For this review, take the finished solid that the model builds, in its own axes (mm). A direction names the side the tool comes from. Round coordinates to 2 decimals unless told otherwise and drop trailing zeros. Order: outer loops, then holes, each group sorted by start corner. A loop starts at its lowest first (then second) coordinate and runs counter-clockwise, first axis right, second up. Notation, with made-up numbers: (30, 52) -> (43, 52) arc R28 cw to (43, 72) -> close; hole circle Ø5 at (16.25, 14.5). An arc over 180 degrees is marked (long way). Answer in a Markdown table with one row per item.
Autodesk Inventor part; units mm, degrees
ref_plane "YZ Plane" through (0, 0, 0) normal (1, 0, 0) x (0, 1, 0)
ref_plane "XZ Plane" through (0, 0, 0) normal (0, 1, 0) x (-1, 0, 0)
ref_plane "XY Plane" through (0, 0, 0) normal (0, 0, 1) x (1, 0, 0)
sketch "Esboço1" plane through (0, 0, 0) normal (0, 1, 0) x (-1, 0, 0)
  circle A0 centre (0, 0) radius 1.5
  dimension "d0" = 3
extrude "Extrusão1" add sketch "Esboço1" along normal blind 10.8
sketch "Esboço2" plane through (0, 10.8, 0) normal (0, 1, 0) x (1, 0, 0)
  circle A0 centre (0, 0) radius 1.5
  arc A1 (1.118, 1) -> (-1.118, 1) centre (0, 0) ccw
  line L0 (-1.118, 1) -> (1.118, 1)
  dimension "d3" = 0.5
extrude "Extrusão2" cut sketch "Esboço2" against normal blind 9 contours L0 A0 picked at (-0.0599, 1.1631)
sketch "Esboço3" plane through (0, 0, 0) normal (0, -1, 0) x (1, 0, 0)
  circle A0 centre (0, 0) radius 0.5
  dimension "d6" = 1
extrude "Extrusão3" add sketch "Esboço3" along normal blind 5
sketch "Esboço4" plane through (0, -5, 0) normal (0, -1, 0) x (1, 0, 0)
  circle A0 centre (0, 0) radius 0.6
  dimension "d9" = 1.2
extrude "Extrusão4" add sketch "Esboço4" along normal blind 0.2
fillet "Arredondamento1" radius 0.2 2 edges at (-1.4013, 10.8, -0.5352) (0.5352, 10.8, 1.4013)
properties part number "Eixo - Encaixe D"
Q1. Take a section at D-D, the plane y = 6.75. Write out the cut boundary in (x, z).
Answer key:
| item | result |
|---|---|
| outline | (-1.12, -1) -> (1.12, -1) arc R1.5 ccw (long way) to start |
Q2. Tool access review of faces 1 (the face through (0, 10.8, 0)), 2 (the face through (0, 6, -1)), 3 (the face through (-0.108, -2.465, 0.488)): name each direction out of +Z, -Z, +X, -X, +Y, -Y from which nothing blocks a thin tool from reaching the whole face with its end or side.
Answer key:
| item | result |
|---|---|
| face 1 | +Z, -Z, +X, -X, +Y |
| face 2 | -Z, +X, -X, +Y |
| face 3 | none |
Q3. Take a section at A-A, the plane z = 0. Write out the cut boundary in (x, y).
Answer key:
| item | result |
|---|---|
| outline | (-1.5, 0) -> (-0.5, 0) -> (-0.5, -5) -> (-0.6, -5) -> (-0.6, -5.2) -> (0.6, -5.2) -> (0.6, -5) -> (0.5, -5) -> (0.5, 0) -> (1.5, 0) -> (1.5, 10.6) arc R0.2 ccw to (1.3, 10.8) -> (-1.3, 10.8) arc R0.2 ccw to (-1.5, 10.6) -> close |
Q4. Clearance check with flat-ended pins moving along their axes: pin 1 Ø0.7 at (x, y) = (-0.5, 5) entering from -Z; pin 2 Ø1.5 at (x, y) = (0.5, -1.5) entering from -Z; pin 3 Ø1 at (y, z) = (7.5, -0.5) entering from +X. State where each tip first meets the part, or that it passes through.
Answer key:
| item | result |
|---|---|
| pin 1 | stops at z = -1 |
| pin 2 | stops at z = -0.5 |
| pin 3 | stops at x = 1.5 |
Q5. Take a section at B-B, the plane x = 0. Write out the cut boundary in (y, z), then the cut area to 3 significant figures.
Answer key:
| item | result |
|---|---|
| outline | (-5.2, -0.6) -> (-5, -0.6) -> (-5, -0.5) -> (0, -0.5) -> (0, -1.5) -> (1.8, -1.5) -> (1.8, -1) -> (10.8, -1) -> (10.8, 1.3) arc R0.2 ccw to (10.6, 1.5) -> (0, 1.5) -> (0, 0.5) -> (-5, 0.5) -> (-5, 0.6) -> (-5.2, 0.6) -> close |
| area | 33.1 mm^2 |
Q6. Take a section at C-C, the plane y = 1. Write out the cut boundary in (x, z), then the cut area to 3 significant figures.
Answer key:
| item | result |
|---|---|
| outline | circle Ø3 at (0, 0) |
| area | 7.07 mm^2 |
Q7. To check wall thickness, follow probe 1 along Y at (x, z) = (-0.35, -1.05); probe 2 along Y at (x, z) = (-0.7, 0.25); probe 3 along Z at (x, y) = (0.75, 3.25). State the ranges of each line that lie inside material, in increasing order.
Answer key:
| item | result |
|---|---|
| probe 1 | y = 0 to 1.8 |
| probe 2 | y = 0 to 10.8 |
| probe 3 | z = -1 to 1.3 |
